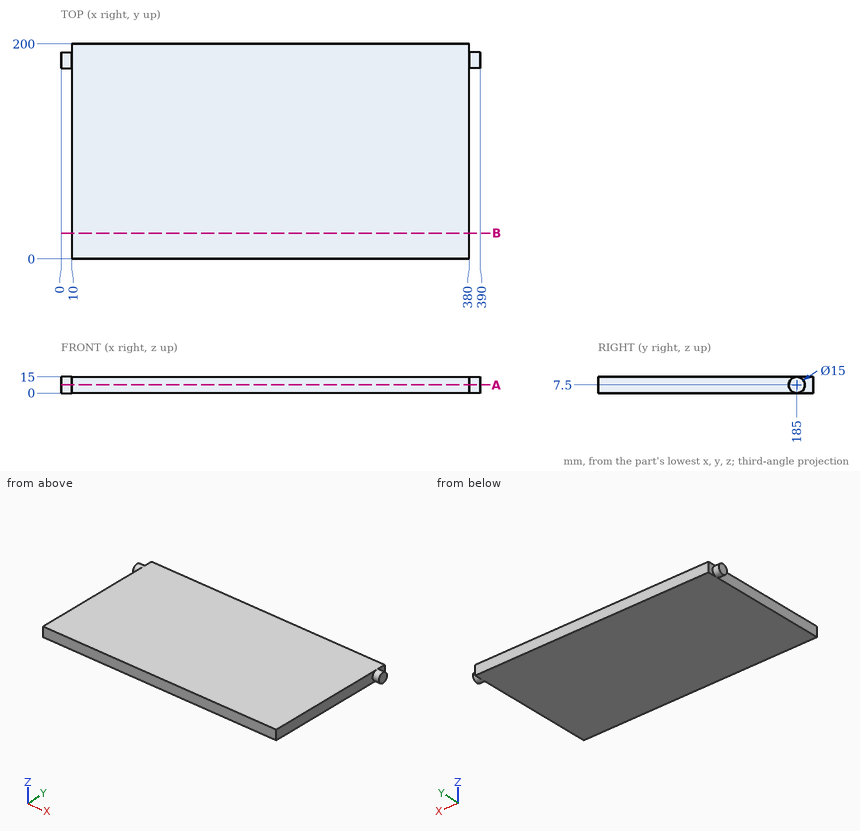
Can you work these out from the drawing? Everything is in mm from the part's minimum corner. Round coordinates to 2 decimals unless told otherwise and drop trailing zeros. Write each loop counter-clockwise with the first axis right and the second up, starting at its lowest first coordinate (ties: lowest second). Pieces come first, ordered by that corner, then holes.
1. Will these pins go through, and if not, where does the flat tip stop? pin 1 Ø10 at (x, y) = (95.5, 21.5) entering from -Z; pin 2 Ø4.5 at (y, z) = (195.5, 10.5) entering from -X.
2. I need wall thicknesses on L1, parallel to X at y = 37, z = 5. Which ranges of the line are inside material? Lowest first, please.
3. Suppose I cut it at A-A (z = 7.5). List the corners of the cut face in (x, y) for me, and give its area (3 significant figures).
4. Suppose I cut it at B-B (y = 24). List the corners of the cut face in (x, z) for me.
Answer sheet:
1. pin 1: stops at z = 0
1. pin 2: stops at x = 10
2. L1: x = 10 to 380
3. outline: (0, 177.5) - (10, 177.5) - (10, 0) - (380, 0) - (380, 177.5) - (390, 177.5) - (390, 192.5) - (380, 192.5) - (380, 200) - (10, 200) - (10, 192.5) - (0, 192.5) - close
3. area: 74,300 mm2
4. outline: (10, 0) - (380, 0) - (380, 15) - (10, 15) - close
